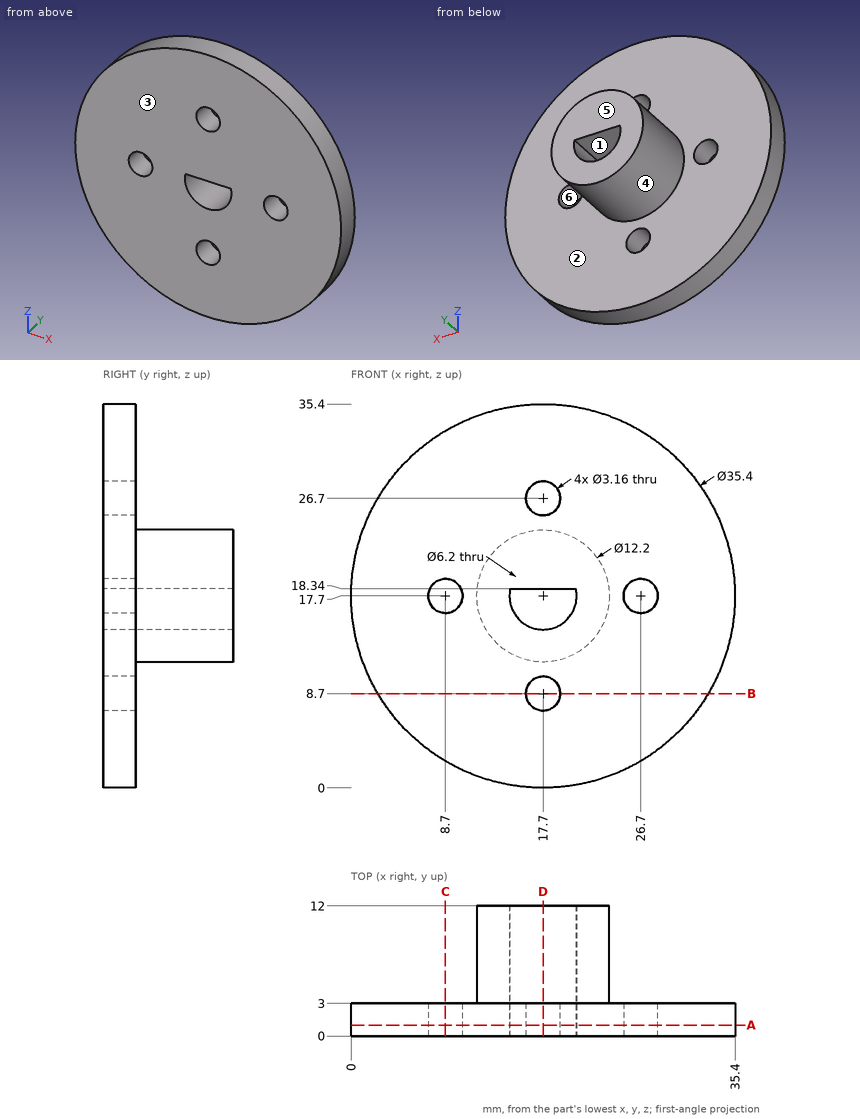
The figure shows three views and two pictorial views of one solid part (mm, origin at its lowest corner). Answer the questions. A direction names the side the tool comes from. Give positions to 0.01 mm unless a question says otherwise; leave off trailing zeros. Write each loop counter-clockwise with the first axis right and the second up, starting at its lowest first coordinate (ties: lowest second). Pieces come first, ordered by that corner, then holes. Notation, with made-up numbers: (67, 5) - (77, 5) arc R30 ccw to (77, 39) - close; hole circle Ø6 at (59, 19.5). An arc over 180 degrees is marked (long way). Return JSON: item names as keys, results as strings.
Q1. For a pull along X with two mould halves and no side action, classify the marked faces 4, 5 and 6 as released by +X, released by -X, zero draft, split by the parting line, or undercut.
Reply:
{"face 4": "split by the parting line", "face 5": "zero draft", "face 6": "undercut"}
Q2. A cutting plane is placed at C-C, the plane x = 8.7. Determine the outline of the cut face in (y, z), and give its area (3 significant figures).
Reply:
{"outline": "(0, 2.46) - (3, 2.46) - (3, 16.12) - (0, 16.12) - close; (0, 19.28) - (3, 19.28) - (3, 32.94) - (0, 32.94) - close", "area": "82.0 mm²"}
Q3. A cutting plane is placed at D-D, the plane x = 17.7. Determine the outline of the cut face in (y, z).
Reply:
{"outline": "(0, 0) - (3, 0) - (3, 7.12) - (0, 7.12) - close; (0, 10.28) - (3, 10.28) - (3, 11.6) - (12, 11.6) - (12, 14.6) - (0, 14.6) - close; (0, 18.34) - (12, 18.34) - (12, 23.8) - (3, 23.8) - (3, 25.12) - (0, 25.12) - close; (0, 28.28) - (3, 28.28) - (3, 35.4) - (0, 35.4) - close"}
Q4. Given P1, Ø3, axis at x = 8.7, z = 17.7, coming from the -Y side; P2, Ø1.5, axis at x = 22.5, y = 8.5, coming from the -Z side; P3, Ø3, axis at y = 4, z = 16, coming from the +X side; P4, Ø6, axis at y = 3, z = 7, coming from the +X side, each flat-ended and moving along its own axis, determine where each tip first touches the part or whether it passes through.
Reply:
{"P1": "through", "P2": "z = 13.14", "P3": "x = 35.39", "P4": "x = 33.64"}
Q5. A cutting plane is placed at B-B, the plane z = 8.7. Determine the outline of the cut face in (x, y).
Reply:
{"outline": "(2.46, 0) - (16.12, 0) - (16.12, 3) - (2.46, 3) - close; (19.28, 0) - (32.94, 0) - (32.94, 3) - (19.28, 3) - close"}
Q6. For the marked faces 1, 2 and 3, determine the directions among +Z, -Z, +X, -X, +Y, -Y from which every point of the face is accessible in a straight line to the end or side of a thin tool.
Reply:
{"face 1": "+Y, -Y", "face 2": "+Y", "face 3": "+Z, -Z, +X, -X, -Y"}
Q7. A cutting plane is placed at A-A, the plane y = 1. Determine the outline of the cut face in (x, z).
Reply:
{"outline": "circle Ø35.4 at (17.7, 17.7); hole circle Ø3.16 at (8.7, 17.7); hole (14.67, 18.34) arc R3.1 ccw (long way) to (20.73, 18.34) - close; hole circle Ø3.16 at (17.7, 8.7); hole circle Ø3.16 at (17.7, 26.7); hole circle Ø3.16 at (26.7, 17.7)"}
Q8. Consider line 1 along Y through (x, z) = (32.5, 13); line 2 along X through (y, z) = (1.5, 19); line 3 along X through (y, z) = (7.5, 17.7). Determine where each line is inside the solid, lowest interval first. Write a range as [from, to].
Reply:
{"line 1": "[0, 3]", "line 2": "[0.05, 7.8], [9.6, 25.8], [27.6, 35.35]", "line 3": "[11.6, 14.6], [20.8, 23.8]"}
